Answer from the drawing. Dimensions are ordinates in mm from the lowest x, y and z of the part. A direction names the side the tool comes from. Give positions to 0.01 mm unless a question says otherwise; leave off trailing zeros. Loops run counter-clockwise (first coordinate to the right, second up) from the corner with the lowest first, then second, coordinate; pieces in that order, holes last. Notation, with made-up numbers: (78.25, 39) - (116.25, 39) arc R26 ccw to (116.25, 65) - close; hole circle Ø9 at (26.5, 11). An arc over 180 degrees is marked (long way). One line per question, with ' | ' between items. Start each with the question number.
1. For a pull along X with two mould halves and no side action, classify the marked faces 3 and 4 as released by +X, released by -X, zero draft, split by the parting line, or undercut.
2. Section A-A (y = 105.5) is taken. Determine the outline of the cut face in (x, z), plus the area to 3 significant figures.
3. Each of these flat-tipped pins is pushed along its axis until it touches: pin 1 (1.5 mm diameter, centred on x = 35, z = 9, fed in from -Y); pin 2 (1 mm diameter, centred on x = 35, z = 5, fed in from +Y) (3 decimals). Where does it stop, or does it pass through?
4. Which of the six approach directions +Z, -Z, +X, -X, +Y, -Y give full straight-line access (tool end or side, diameter ignored) to the marked faces 1 and 2?
5. Section D-D (x = 50) is taken. Determine the outline of the cut face in (y, z), plus the area to 3 significant figures.
6. Section C-C (y = 43) is taken. Determine the outline of the cut face in (x, z), plus the area to 3 significant figures.
7. Find the intervals of material crossed by line 1 (X direction, y = 91, z = 8.75); line 2 (X direction, y = 31.5, z = 8.5) (1 decimal); line 3 (Y direction, x = 19, z = 3.5), in increasing order.
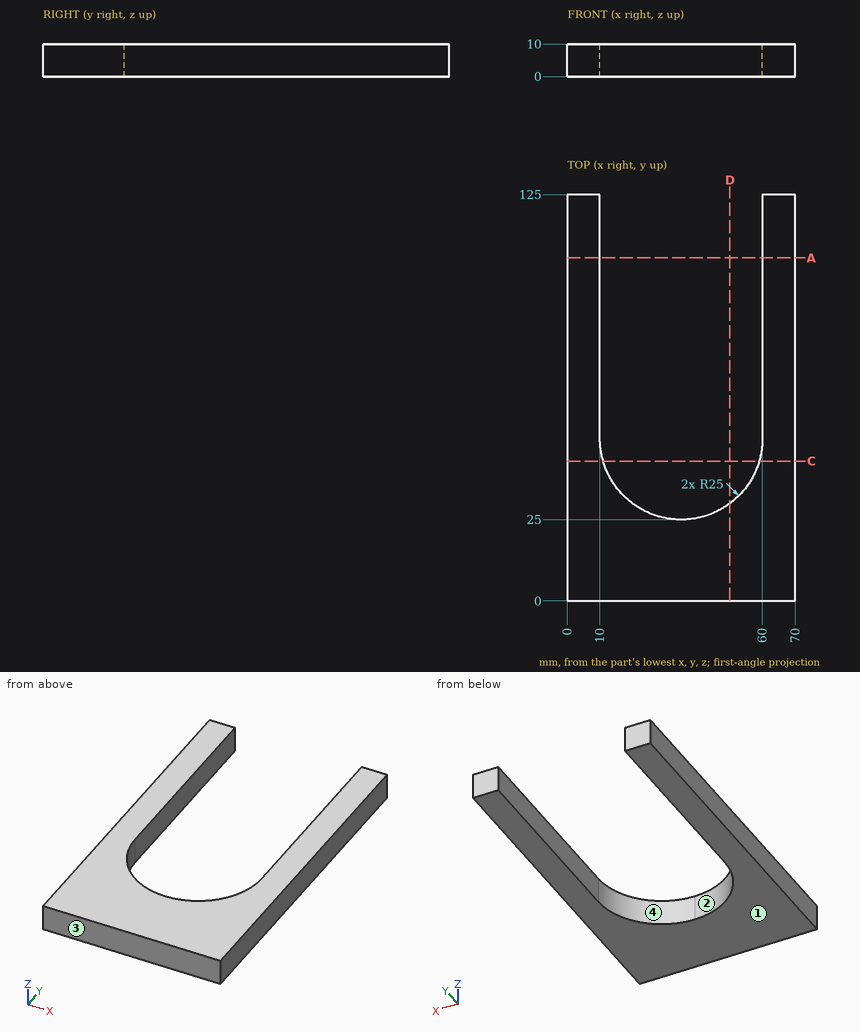
Conclusion:
1) face 3: zero draft | face 4: undercut
2) outline: (0, 0) - (10, 0) - (10, 10) - (0, 10) - close; (60, 0) - (70, 0) - (70, 10) - (60, 10) - close | area: 200 mm²
3) pin 1: y = 0 | pin 2: y = 25.005
4) face 1: -Z, +X, -X, +Y, -Y | face 2: +Z, -Z, +Y
5) outline: (0, 0) - (30, 0) - (30, 10) - (0, 10) - close | area: 300 mm²
6) outline: (0, 0) - (11, 0) - (11, 10) - (0, 10) - close; (59, 0) - (70, 0) - (70, 10) - (59, 10) - close | area: 220 mm²
7) line 1: 0 to 10, 60 to 70 | line 2: 0 to 18.2, 51.8 to 70 | line 3: 0 to 30.79
